Autodesk Inventor part; units mm, degrees
ref_plane "YZ Plane" through (0, 0, 0) normal (1, 0, 0) x (0, 1, 0)
ref_plane "XZ Plane" through (0, 0, 0) normal (0, 1, 0) x (-1, 0, 0)
ref_plane "XY Plane" through (0, 0, 0) normal (0, 0, 1) x (1, 0, 0)
sketch "Esboço1" plane through (0, 0, 0) normal (1, 0, 0) x (0, 1, 0)
  line L0 (0, 0) -> (50.8, 0)
  line L1 (50.8, 0) -> (50.8, -86.2)
  line L2 (50.8, -86.2) -> (0, -86.2)
  line L3 (0, -86.2) -> (0, 0)
  circle A0 centre (38.1, -5) radius 2.5
  circle A1 centre (25.4, -5) radius 2.5
  circle A2 centre (12.7, -5) radius 2.5
  circle A3 centre (38.1, -17.7) radius 2.5
  circle A4 centre (25.4, -17.7) radius 2.5
  circle A5 centre (12.7, -17.7) radius 2.5
  circle A6 centre (38.1, -30.4) radius 2.5
  circle A7 centre (25.4, -30.4) radius 2.5
  circle A8 centre (12.7, -30.4) radius 2.5
  circle A9 centre (38.1, -43.1) radius 2.5
  circle A10 centre (25.4, -43.1) radius 2.5
  circle A11 centre (12.7, -43.1) radius 2.5
  circle A12 centre (38.1, -55.8) radius 2.5
  circle A13 centre (25.4, -55.8) radius 2.5
  circle A14 centre (12.7, -55.8) radius 2.5
  circle A15 centre (38.1, -68.5) radius 2.5
  circle A16 centre (25.4, -68.5) radius 2.5
  circle A17 centre (12.7, -68.5) radius 2.5
  circle A18 centre (38.1, -81.2) radius 2.5
  circle A19 centre (25.4, -81.2) radius 2.5
  circle A20 centre (12.7, -81.2) radius 2.5
  dimension "d0" = 50.8
  dimension "d1" = 86.2
  dimension "d2" = 5
  dimension "d3" = 5
  dimension "d4" = 5
  dimension "d5" = 5
  dimension "d6" = 5
  dimension "d7" = 5
  dimension "d8" = 12.7
  dimension "d9" = 12.7
  dimension "d10" = 12.7
  dimension "d13" = 12.7
extrude "Extrusão1" add sketch "Esboço1" along normal blind 5
sketch "Esboço2" plane through (0, 0, 0) normal (-1, 0, 0) x (0, 0, 1)
  line L0 (-86.2, 0) -> (-149.7, 0)
  line L1 (-149.7, 0) -> (-149.7, 50.8)
  line L2 (-149.7, 50.8) -> (-86.2, 50.8)
  line L3 (-86.2, 50.8) -> (-86.2, 0)
  circle A0 centre (-144.7, 38.1) radius 2.5
  circle A1 centre (-144.7, 25.4) radius 2.5
  circle A2 centre (-144.7, 12.7) radius 2.5
  circle A3 centre (-132, 12.7) radius 2.5
  circle A4 centre (-132, 25.4) radius 2.5
  circle A5 centre (-132, 38.1) radius 2.5
  circle A6 centre (-119.3, 38.1) radius 2.5
  circle A7 centre (-119.3, 25.4) radius 2.5
  circle A8 centre (-119.3, 12.7) radius 2.5
  circle A9 centre (-106.6, 12.7) radius 2.5
  circle A10 centre (-93.9, 12.7) radius 2.5
  circle A11 centre (-93.9, 25.4) radius 2.5
  circle A12 centre (-106.6, 25.4) radius 2.5
  circle A13 centre (-106.6, 38.1) radius 2.5
  circle A14 centre (-93.9, 38.1) radius 2.5
  point P0 (0, 0)
  dimension "d20" = 50.8
  dimension "d21" = 5
extrude "Extrusão2" add sketch "Esboço2" against normal blind 5
sketch "Esboço3" plane through (0, 0, 0) normal (-1, 0, 0) x (0, 0, 1)
  circle A0 centre (-121.1, 85.9607) radius 4.5847
  circle A1 centre (63.725, 144.496) radius 17.5
  circle A2 centre (51.025, 169.896) radius 2.5
  circle A3 centre (76.425, 169.896) radius 2.5
  circle A4 centre (76.425, 119.096) radius 2.5
  circle A5 centre (51.025, 119.096) radius 2.5
  circle A6 centre (-121.1, 85.9607) radius 14.25
  circle A7 centre (63.725, 144.496) radius 20
  line L0 (-149.7, 50.8) -> (0, 50.8)
  line L1 (-149.7, 50.8) -> (-149.7, 85.9607)
  arc A8 (86.0063, 114.3333) -> (50.7735, 179.6885) centre (63.725, 144.496) ccw
  arc A9 (-130.9776, 112.8008) -> (-149.7, 85.9607) centre (-121.1, 85.9607) ccw
  line L2 (50.7735, 179.6885) -> (-130.9776, 112.8008)
  line L3 (0, 50.8) -> (0, 0)
  line L4 (0, 50.8) -> (86.0063, 114.3333)
  dimension "d26" = 28.5
  dimension "d27" = 40
  dimension "d28" = 75
extrude "Extrusão3" add sketch "Esboço3" against normal blind 5 contours L1 A9 L2 A8 L4 L0
fillet "Arredondamento1" radius 5 3 edges at (2.5, 50.8, 0) (2.5, 0, 0) (2.5, 0, -149.7)
sketch "Esboço4" plane through (0, 0, 0) normal (-1, 0, 0) x (0, 0, 1)
  circle A0 centre (-121.1, 85.9607) radius 14.25
  point P0 (0, 0)
extrude "Extrusão4" add sketch "Esboço4" against normal blind 5
equation "\"d6\" = d5"
equation "\"d7\" = d6"
equation "\"d9\" = d8"
equation "\"d10\" = d9"
properties part number "CHAPA FIXAÇÃO DIREITA 1 V2"
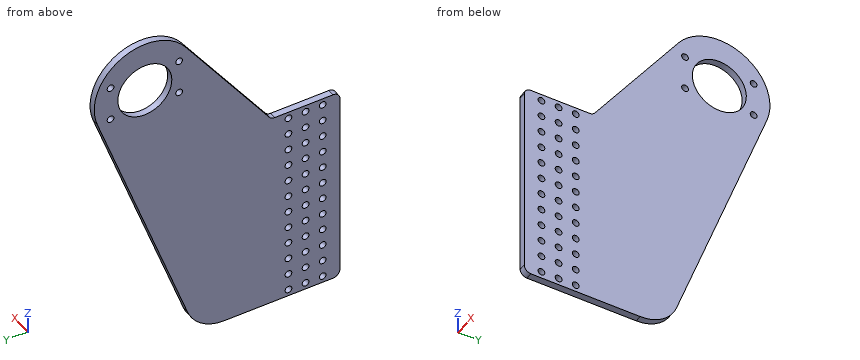
Could you check a few things on this model? Use its own coordinates, in mm. Round coordinates to 2 decimals unless told otherwise and drop trailing zeros. Write each loop counter-clockwise with the first axis right and the second up, starting at its lowest first coordinate (ties: lowest second). Pieces come first, ordered by that corner, then holes. Notation, with made-up numbers: M 84,-1.75 L 125,-1.75 A29 cw 125,21.25 Z; hole C 9,31 d2. An arc over 180 degrees is marked long. Answer in a Markdown table with one row per item. Add a question column.
Q1. Imagine slicing it at B-B (z = 66.5). Please give me the cut outline in (x, y), then the cut area to 3 significant figures.
Q2. If I drill on line 1 (Y direction, x = 1.5, z = -106.6); line 2 (Y direction, x = 2, z = -55.5); line 3 (Z direction, x = 4.75, y = 33), over which ranges is the centre line in solid material (lowest first)? Write a range as from..to.
Q3. Imagine slicing it at C-C (z = -119.3). Please give me the cut outline in (x, y).
Q4. Will these pins go through, and if not, where does the flat tip stop? pin 1 Ø2 at (y, z) = (40, -123) entering from -X; pin 2 Ø2.5 at (x, y) = (2, 20) entering from +Z; pin 3 Ø2 at (x, z) = (4.5, 26.5) entering from -Y; pin 4 Ø1.5 at (x, z) = (2, 62) entering from +Y.
Q5. Imagine slicing it at A-A (y = 151.5). Please give me the cut outline in (x, z), then the cut area to 3 significant figures.
Q6. Imagine slicing it at D-D (y = 25.4). Give the number of separate pieces and of enclosed holes in the cut face, then the cut area to 4 significant figures.
Values:
| question | item | result |
|---|---|---|
| 1 | outline | M 0,99.92 L 5,99.92 L 5,124.69 L 0,124.69 Z; M 0,164.3 L 5,164.3 L 5,181.89 L 0,181.89 Z |
| 1 | area | 212 mm^2 |
| 2 | line 1 | 0..10.2, 15.2..22.9, 27.9..35.6, 40.6..121.77 |
| 2 | line 2 | 0..10.22, 15.18..22.92, 27.88..35.62, 40.58..140.58 |
| 2 | line 3 | -149.7..0 |
| 3 | outline | M 0,0 L 5,0 L 5,10.2 L 0,10.2 Z; M 0,15.2 L 5,15.2 L 5,22.9 L 0,22.9 Z; M 0,27.9 L 5,27.9 L 5,35.6 L 0,35.6 Z; M 0,40.6 L 5,40.6 L 5,117.1 L 0,117.1 Z |
| 4 | pin 1 | x = 0 |
| 4 | pin 2 | z = 0 |
| 4 | pin 3 | y = 69.64 |
| 4 | pin 4 | y = 181.98 |
| 5 | outline | M 0,-25.82 L 5,-25.82 L 5,44.99 L 0,44.99 Z; M 0,82.46 L 5,82.46 L 5,100.57 L 0,100.57 Z |
| 5 | area | 445 mm^2 |
| 6 | separate pieces | 13 |
| 6 | enclosed holes | 0 |
| 6 | area | 448.5 mm^2 |
